```python
from build123d import *

# Parameters (mm, degrees)
SKETCH1_R                = 9
BOSS_EXTRUDE1_DEPTH      = 15
BOSS_EXTRUDE2_DEPTH      = 63.5
BOSS_EXTRUDE2_DEPTH_BACK = 63.5
CUT_EXTRUDE1_DEPTH       = 200
CUT_EXTRUDE1_DEPTH_BACK  = 200
SKETCH4_W                = 5
SKETCH4_H                = 40


with BuildPart() as part:
    # Sketch1 → Boss-Extrude1 (new body)
    with BuildSketch(Plane(origin=(0, 0, 0), x_dir=(1, 0, 0), z_dir=(0, 1, 0))):
        with BuildLine():
            Line((-115, 211.991055507), (-115, -205))
            ThreePointArc((-115, -205), (-109.142135624, -219.142135624), (-95, -225))
            Line((-95, -225), (95, -225))
            ThreePointArc((95, -225), (109.142135624, -219.142135624), (115, -205))
            Line((115, -205), (115, 211.991055507))
            ThreePointArc((115, 211.991055507), (111.765445383, 222.896092926), (103.108015888, 230.273836432))
            Line((103.108015888, 230.273836432), (8.108015888, 272.404271215))
            ThreePointArc((8.108015888, 272.404271215), (0, 274.12149029), (-8.108015888, 272.404271215))
            Line((-8.108015888, 272.404271215), (-103.108015888, 230.273836432))
            ThreePointArc((-103.108015888, 230.273836432), (-111.765445383, 222.896092926), (-115, 211.991055507))
        make_face()
        with Locations(Location((0, 254.12149029, 0), (0, 0, 270))):
            Circle(SKETCH1_R, mode=Mode.SUBTRACT)
    extrude(amount=BOSS_EXTRUDE1_DEPTH)

    # Sketch2 → Boss-Extrude2 (add, two sides: drawn at the far end of the back side and taken through both)
    with BuildSketch(Plane(origin=(0, 0, 0), x_dir=(0, 0, -1), z_dir=(1, 0, 0)).offset(-BOSS_EXTRUDE2_DEPTH_BACK)):
        Polygon((-160, 15), (-160, 65), (90, 65), (140, 15), align=None)
    extrude(amount=BOSS_EXTRUDE2_DEPTH + BOSS_EXTRUDE2_DEPTH_BACK)

    # Sketch4 → Cut-Extrude1 (cut, two sides: drawn at the far end of the back side and taken through both)
    with BuildSketch(Plane.XY.offset(-CUT_EXTRUDE1_DEPTH_BACK)):
        with Locations((-50, 35)):
            Rectangle(SKETCH4_W, SKETCH4_H)
        with Locations((50, 35)):
            Rectangle(SKETCH4_W, SKETCH4_H)
        with Locations((30, 35)):
            Rectangle(SKETCH4_W, SKETCH4_H)
        with Locations((10, 35)):
            Rectangle(SKETCH4_W, SKETCH4_H)
        with Locations((-10, 35)):
            Rectangle(SKETCH4_W, SKETCH4_H)
        with Locations((-30, 35)):
            Rectangle(SKETCH4_W, SKETCH4_H)
    extrude(amount=CUT_EXTRUDE1_DEPTH + CUT_EXTRUDE1_DEPTH_BACK, mode=Mode.SUBTRACT)


solid = part.part
```
Geometry: final body of the model. Coordinates: model frame, mm. A direction names the side the tool comes from. Round coordinates to 2 decimals unless told otherwise and drop trailing zeros. Order: outer loops, then holes, each group sorted by start corner. A loop starts at its lowest first (then second) coordinate and runs counter-clockwise, first axis right, second up. Notation, with made-up numbers: M -28,-34 L -14,-34 A14 ccw -14,-12 Z; hole C -38.75,36 d6. An arc over 180 degrees is marked long. Use one line per item in the form item = value. Start each with the question number.
Q1. Cut plane B-B (y = 37.5). Return loops of the section in (x, z).
Q2. Access query for faces 1 (the face through (12.5, 35, 8)), 2 (the face through (115, 7, -1)). Directions: +Z, -Z, +X, -X, +Y, -Y. A direction counts if a zero-diameter tool reaches every point of the face in a straight line with its end or side. Return the directions, or none.
Q3. Mould query, pull axis Y, two halves, no side actions, for faces 3 (the face through (-2, 0, -28)), 4 (the face through (47.5, 35, 8)), 5 (the face through (-115, 7, -6)). Classes: +Y half, -Y half, draft (parallel to the pull), parting line (faces both ways), or undercut.
Q4. Pin query (flat end, axial travel): pin 1 Ø4 at (x, y) = (45, 48.5) entering from -Z; pin 2 Ø15 at (y, z) = (40, 56) entering from -X; pin 3 Ø4 at (y, z) = (32, 28) entering from +X. Return the tip coordinate at first contact, or that it passes through.
Q5. Material intervals for line 1 (Y direction, x = -31.5, z = -22); line 2 (Y direction, x = -79, z = 132.5); line 3 (X direction, y = 60.5, z = 11), sorted ascending. Write a range as [from, to].
Q6. Cut plane A-A (x = 0). Return loops of the section in (y, z), and give its area (3 significant figures).
Q7. Cut plane C-C (z = -59). Count the separate pieces of the cut face and the enclosed holes in it, and give its area (3 significant figures).
Q8. Cut plane D-D (z = -188.5). Return loops of the section in (x, y).
Geometry results:
q1.outline = M -63.5,-117.5 L -52.5,-117.5 L -52.5,160 L -63.5,160 Z; M -47.5,-117.5 L -32.5,-117.5 L -32.5,160 L -47.5,160 Z; M -27.5,-117.5 L -12.5,-117.5 L -12.5,160 L -27.5,160 Z; M -7.5,-117.5 L 7.5,-117.5 L 7.5,160 L -7.5,160 Z; M 12.5,-117.5 L 27.5,-117.5 L 27.5,160 L 12.5,160 Z; M 32.5,-117.5 L 47.5,-117.5 L 47.5,160 L 32.5,160 Z; M 52.5,-117.5 L 63.5,-117.5 L 63.5,160 L 52.5,160 Z
q2.face_1 = +Z, -Z
q2.face_2 = +Z, -Z, +X, +Y, -Y
q3.face_3 = -Y half
q3.face_4 = undercut
q3.face_5 = draft
q4.pin_1 = -108.5
q4.pin_2 = -63.5
q4.pin_3 = 63.5
q5.line_1 = [0, 15], [55, 65]
q5.line_2 = [0, 15]
q5.line_3 = [-63.5, 63.5]
q6.outline = M 0,-274.12 L 15,-274.12 L 15,-263.12 L 0,-263.12 Z; M 0,-245.12 L 15,-245.12 L 15,-140 L 65,-90 L 65,160 L 15,160 L 15,225 L 0,225 Z
q6.area = 21,000 mm^2
q7.separate_pieces = 1
q7.enclosed_holes = 6
q7.area = 8,600 mm^2
q8.outline = M -115,0 L 115,0 L 115,15 L -115,15 Z
